Can you work these out from the drawing? Everything is in mm from the part's minimum corner. A direction names the side the tool comes from. Round coordinates to 2 decimals unless told otherwise and drop trailing zeros. Write each loop counter-clockwise with the first axis right and the second up, starting at its lowest first coordinate (ties: lowest second). Pieces come first, ordered by that corner, then holes. Notation, with made-up numbers: (19, 78.25) -> (26, 78.25) arc R13 ccw to (26, 95.25) -> close; hole circle Ø7 at (23.25, 74). An arc over 180 degrees is marked (long way). Put each result on its own line as item: value. Start each with the question number.
1. I need wall thicknesses on probe 1 along Z at (x, y) = (3.5, 25.5) (1 decimal). Which ranges of the line are inside material? Lowest first, please. Write a range as from..to.
2. For pin 1 (4.5 mm diameter, centred on x = 7.62, y = 10.16, fed in from -Z); pin 2 (12 mm diameter, centred on x = 14.5, y = 16.5, fed in from +Z) (3 decimals); pin 3 (10 mm diameter, centred on x = 22.5, z = 16.5, fed in from +Y) (3 decimals), each with a flat end and sliding along its axis, tell me the tip position at first contact or that it passes through.
3. Suppose I cut it at B-B (y = 10.16). Please give me the cut outline in (x, z) (1 decimal).
4. Suppose I cut it at A-A (x = 17.78). Count the separate pieces of the cut face and the enclosed holes in it.
5. Suppose I cut it at D-D (y = 5.75). Please give me the cut outline in (x, z) (1 decimal).
6. Suppose I cut it at C-C (z = 2). Please give me the cut outline in (x, y) (1 decimal).
7. Which directions (+Z, -Z, +X, -X, +Y, -Y) give clear straight access to the entire face, cutting with the end or side of a thin tool? Please do the marked faces 1 and 2.
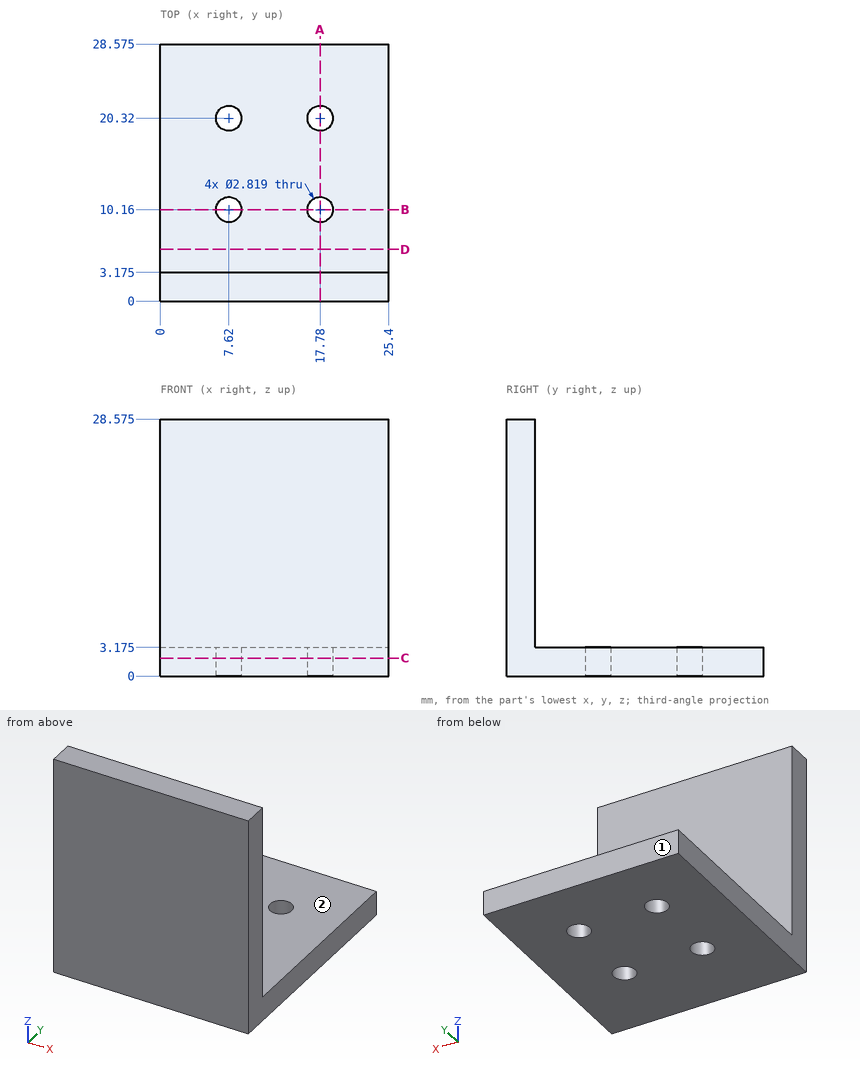
Verdict:
1. probe 1: z = 0..3.2
2. pin 1: stops at z = 0
2. pin 2: stops at z = 3.175
2. pin 3: stops at y = 3.175
3. outline: (0, 0) -> (6.2, 0) -> (6.2, 3.2) -> (0, 3.2) -> close; (9, 0) -> (16.4, 0) -> (16.4, 3.2) -> (9, 3.2) -> close; (19.2, 0) -> (25.4, 0) -> (25.4, 3.2) -> (19.2, 3.2) -> close
4. separate pieces: 3
4. enclosed holes: 0
5. outline: (0, 0) -> (25.4, 0) -> (25.4, 3.2) -> (0, 3.2) -> close
6. outline: (0, 0) -> (25.4, 0) -> (25.4, 28.6) -> (0, 28.6) -> close; hole circle Ø2.8 at (7.6, 10.2); hole circle Ø2.8 at (7.6, 20.3); hole circle Ø2.8 at (17.8, 10.2); hole circle Ø2.8 at (17.8, 20.3)
7. face 1: +Z, -Z, +X, -X, +Y
7. face 2: +Z, +X, -X, +Y
